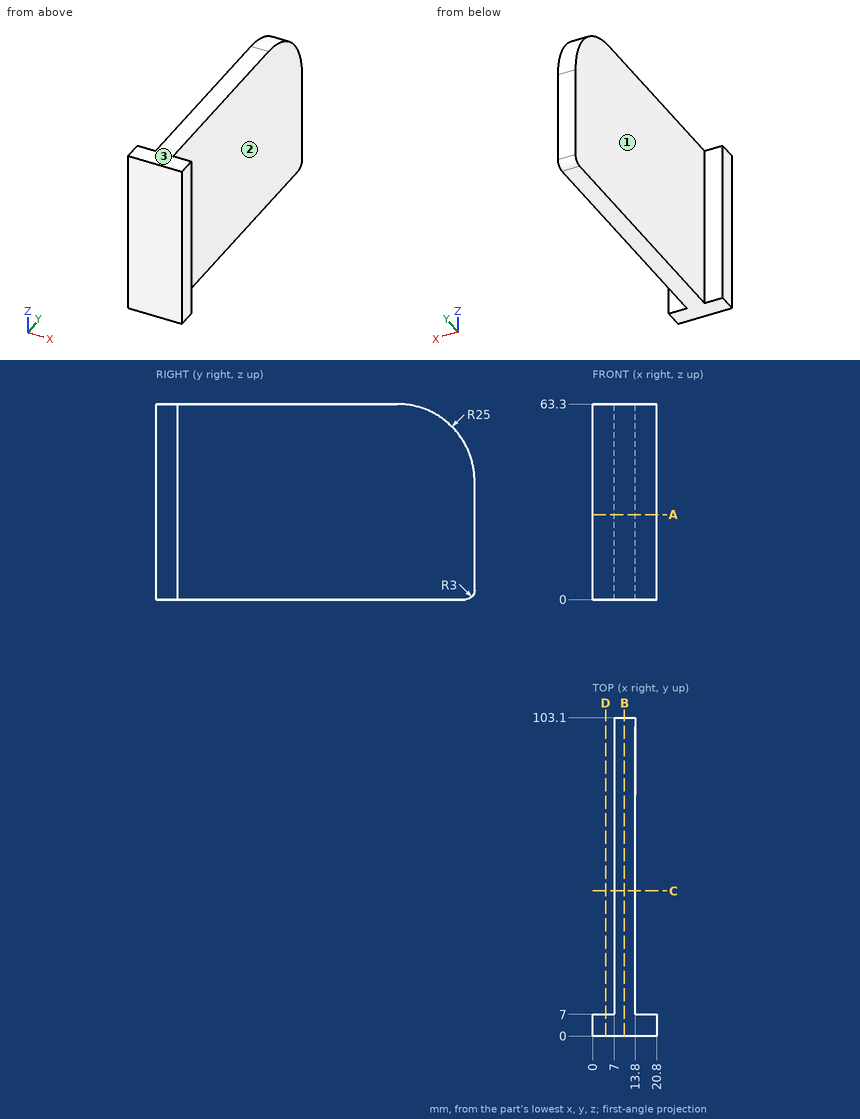
The drawing under review shows one solid part. Ordinate dimensions are in mm from its lowest x, y, z. A direction names the side the tool comes from. Coordinates: 2 decimals unless noted, no trailing zeros. Loops run counter-clockwise (first coordinate to the right, second up) from the corner with the lowest first, then second, coordinate; pieces in that order, holes last. Notation, with made-up numbers: (-4.5, 80.5) - (39.5, 80.5) arc R34 cw to (39.5, 110.5) - close; hole circle Ø2 at (60, 38.25). An arc over 180 degrees is marked (long way). Return JSON: item names as keys, results as strings.
Item 1: Take a section at C-C (y = 47). Give the boundary of the cut face in (x, z), then the cut area to 3 significant figures.
Determined:
{"outline": "(7, 0) - (13.8, 0) - (13.8, 63.3) - (7, 63.3) - close", "area": "430 mm2"}
Item 2: Take a section at A-A (z = 27.5). Give the boundary of the cut face in (x, y).
Determined:
{"outline": "(0, 0) - (20.8, 0) - (20.8, 7) - (13.8, 7) - (13.8, 103.1) - (7, 103.1) - (7, 7) - (0, 7) - close"}
Item 3: Take a section at D-D (x = 4.25). Give the boundary of the cut face in (y, z), then the cut area to 3 significant figures.
Determined:
{"outline": "(0, 0) - (7, 0) - (7, 63.3) - (0, 63.3) - close", "area": "443 mm2"}
Item 4: Take a section at B-B (x = 10.25). Give the boundary of the cut face in (y, z), then the cut area to 3 significant figures.
Determined:
{"outline": "(0, 0) - (100.1, 0) arc R3 ccw to (103.1, 3) - (103.1, 38.3) arc R25 ccw to (78.1, 63.3) - (0, 63.3) - close", "area": "6,390 mm2"}
Item 5: For line 1 (Y direction, x = 1.75, z = 50); line 2 (X direction, y = 52, z = 37.5); line 3 (Y direction, x = 13.75, z = 45.5), list the stretches that pass through material, from the lowest coordinate up.
Determined:
{"line 1": "y = 0 to 7", "line 2": "x = 7 to 13.8", "line 3": "y = 0 to 102.04"}
Item 6: Insertion check: pin 1 (2 mm diameter, centred on x = 4, z = 31.5, fed in from +Y); pin 2 (2 mm diameter, centred on y = 46, z = 9, fed in from -X); pin 3 (4 mm diameter, centred on x = 6, z = 44, fed in from +Y). Each pin has a flat end and moves straight along its axis. Give the tip position at first contact, or say it passes through.
Determined:
{"pin 1": "stops at y = 7", "pin 2": "stops at x = 7", "pin 3": "stops at y = 102.78"}
Item 7: For the marked faces 1, 2 and 3, list the 3-axis set-ups (+Z, -Z, +X, -X, +Y, -Y) from which the entire face can be reached by the end or side of a thin tool; tool diameter is ignored.
Determined:
{"face 1": "+Z, -Z, -X, +Y", "face 2": "+Z, -Z, +X, +Y", "face 3": "+Z, +X, -X, +Y, -Y"}
